```python
from build123d import *
from OCP.BRepFilletAPI import BRepFilletAPI_MakeChamfer

# Parameters (mm, degrees)
SKETCH1_W                = 70
SKETCH1_H                = 150
BOSS_EXTRUDE1_DEPTH      = 5
SKETCH2_W                = 4
SKETCH2_H                = 15
BOSS_EXTRUDE2_DEPTH      = 15
BOSS_EXTRUDE3_REACH      = 89.321
SKETCH3_R                = 3
CHAMFER1_SIZE            = 4
CHAMFER2_SIZE            = 4
CHAMFER3_SIZE            = 4
CHAMFER4_SIZE            = 10
CHAMFER5_SIZE            = 20
SKETCH4_W                = 3
SKETCH4_H                = 10
BOSS_EXTRUDE4_DEPTH      = 10
CHAMFER6_SIZE            = 2
SKETCH5_R                = 1.5
CUT_EXTRUDE1_DEPTH       = 100.969995499
CUT_EXTRUDE2_DEPTH       = 106
BOSS_EXTRUDE5_DEPTH      = 10
BOSS_EXTRUDE5_DEPTH_BACK = 3
SKETCH7_W                = 18
SKETCH7_H                = 2.192346064
CHAMFER7_SIZE            = 3
CHAMFER7_SIZE2           = 3.21710613
FILLET1_R                = 2
SKETCH8_R                = 1.5
CUT_EXTRUDE3_DEPTH       = 10
CHAMFER8_SIZE            = 1
CHAMFER8_SIZE2           = 0.487732589
FILLET2_R                = 1
SKETCH9_W                = 23.659390011
SKETCH9_H                = 22.018276252
CUT_EXTRUDE4_DEPTH       = 20


with BuildPart() as part:
    # Sketch1 → Boss-Extrude1 (new body)
    with BuildSketch(Plane(origin=(0, 0, 0), x_dir=(1, 0, 0), z_dir=(0, 1, 0))):
        Rectangle(SKETCH1_W, SKETCH1_H)
    extrude(amount=BOSS_EXTRUDE1_DEPTH)

    # Sketch2 → Boss-Extrude2 (add)
    with BuildSketch(Plane(origin=(0, 5, 0), x_dir=(1, 0, 0), z_dir=(0, 1, 0))):
        with Locations((-7, 62.5)):
            Rectangle(SKETCH2_W, SKETCH2_H)
        with Locations((7, 62.5)):
            Rectangle(SKETCH2_W, SKETCH2_H)
    extrude(amount=BOSS_EXTRUDE2_DEPTH)

    # Sketch3 → Boss-Extrude3 (add, up to next)
    with BuildSketch(Plane(origin=(-5, 0, 0), x_dir=(0, 0, -1), z_dir=(1, 0, 0)), mode=Mode.PRIVATE) as boss_extrude3_sk1:
        with Locations(Location((62.5, 12.5, 0), (0, 0, 180))):
            Circle(SKETCH3_R)
    boss_extrude3_tool1 = extrude(boss_extrude3_sk1.sketch, amount=BOSS_EXTRUDE3_REACH, mode=Mode.PRIVATE) - part.part
    add(boss_extrude3_tool1.solids().sort_by_distance((-5, 12.5, -62.5))[0])

    # Chamfer1
    chamfer1_edges = [part.edges().sort_by_distance(p)[0] for p in [
        (-7, 20, -70),
        (-7, 20, -55),
        (7, 20, -70),
        (7, 20, -55),
    ]]
    chamfer(chamfer1_edges, length=CHAMFER1_SIZE)

    # Chamfer2
    chamfer2_edges = [part.edges().sort_by_distance(p)[0] for p in [
        (-7, 5, -70),
        (-7, 5, -55),
        (7, 5, -70),
        (7, 5, -55),
    ]]
    chamfer(chamfer2_edges, length=CHAMFER2_SIZE)

    # Chamfer3
    chamfer3_edges = [part.edges().sort_by_distance(p)[0] for p in [
        (9, 5, -62.5),
        (-9, 5, -62.5),
    ]]
    chamfer(chamfer3_edges, length=CHAMFER3_SIZE)

    # Chamfer4
    chamfer4_edges = [part.edges().sort_by_distance(p)[0] for p in [
        (-35, 2.5, -75),
        (35, 2.5, -75),
    ]]
    chamfer(chamfer4_edges, length=CHAMFER4_SIZE)

    # Chamfer5
    chamfer5_edges = [part.edges().sort_by_distance(p)[0] for p in [
        (35, 2.5, 75),
        (-35, 2.5, 75),
    ]]
    chamfer(chamfer5_edges, length=CHAMFER5_SIZE)

    # Sketch4 → Boss-Extrude4 (add)
    with BuildSketch(Plane(origin=(0, 5, 0), x_dir=(1, 0, 0), z_dir=(0, 1, 0))):
        with Locations((26.5, -25)):
            Rectangle(SKETCH4_W, SKETCH4_H)
        with Locations((-26.5, -25)):
            Rectangle(SKETCH4_W, SKETCH4_H)
    extrude(amount=BOSS_EXTRUDE4_DEPTH)

    # Chamfer6
    chamfer6_edges = [part.edges().sort_by_distance(p)[0] for p in [
        (26.5, 15, 20),
        (26.5, 15, 30),
        (-26.5, 15, 20),
        (-26.5, 15, 30),
    ]]
    chamfer(chamfer6_edges, length=CHAMFER6_SIZE)

    # Sketch5 → Cut-Extrude1 (cut, through all)
    with BuildSketch(Plane(origin=(28, 0, 0), x_dir=(0, 0, -1), z_dir=(1, 0, 0))):
        with Locations((-25, 11)):
            Circle(SKETCH5_R)
    extrude(amount=-CUT_EXTRUDE1_DEPTH, mode=Mode.SUBTRACT)

    # Sketch6 → Cut-Extrude2 (cut)
    with BuildSketch(Plane(origin=(35, 0, 0), x_dir=(0, 0, -1), z_dir=(1, 0, 0))):
        Polygon((-75, 5), (44.602239444, 5), (44.602239444, 35.253881219), (84.386815395, 35.253881219), (84.386815395, 5), (84.386815395, -21.159404211), (-75, -21.159404211), align=None)
    extrude(amount=-CUT_EXTRUDE2_DEPTH, mode=Mode.SUBTRACT)


with BuildPart() as cut_extrude2_piece_1:
    # of the separate pieces the step leaves, piece 1, a body of its own (cut_extrude2_pieces)
    add(part.part.solids().sort_by_distance((-25, 13, 20))[0])

    # Sketch9 → Cut-Extrude4 (cut)
    with BuildSketch(Plane(origin=(0, 0, 16), x_dir=(-1, 0, 0), z_dir=(0, 0, -1))):
        with Locations((24.129769204, 9.145253251)):
            Rectangle(SKETCH9_W, SKETCH9_H)
    extrude(amount=-CUT_EXTRUDE4_DEPTH, mode=Mode.SUBTRACT)


with BuildPart() as cut_extrude2_piece_2:
    # of the separate pieces the step leaves, piece 2, a body of its own (cut_extrude2_pieces)
    add(part.part.solids().sort_by_distance((25, 13, 20))[0])

    # Sketch7 → Boss-Extrude5 (add, two sides: drawn at the far end of the back side and taken through both)
    with BuildSketch(Plane(origin=(28, 0, 0), x_dir=(0, 0, -1), z_dir=(1, 0, 0)).offset(-BOSS_EXTRUDE5_DEPTH_BACK)):
        with Locations((-25, 6.096173032)):
            Rectangle(SKETCH7_W, SKETCH7_H)
    extrude(amount=BOSS_EXTRUDE5_DEPTH + BOSS_EXTRUDE5_DEPTH_BACK)

    # Chamfer7: one chamfer whose edges measure the first distance from different faces: ONE call of the kernel's chamfer builder (chamfer() names one face for all edges)
    chamfer7_edges_1 = [cut_extrude2_piece_2.edges().sort_by_distance(p)[0] for p in [
        (25, 6.096173032, 34),
    ]]
    chamfer7_side_1 = [cut_extrude2_piece_2.faces().sort_by_distance(p)[0] for p in [
        (31.5, 6.096173032, 34),
    ]]
    chamfer7_edges_2 = [cut_extrude2_piece_2.edges().sort_by_distance(p)[0] for p in [
        (25, 6.096173032, 16),
    ]]
    chamfer7_side_2 = [cut_extrude2_piece_2.faces().sort_by_distance(p)[0] for p in [
        (25, 9.127734828, 25),
    ]]
    chamfer7 = BRepFilletAPI_MakeChamfer(cut_extrude2_piece_2.part.solid().wrapped)
    for e in chamfer7_edges_1:
        chamfer7.Add(CHAMFER7_SIZE, CHAMFER7_SIZE2, e.wrapped, chamfer7_side_1[0].wrapped)  # the first distance lies on this face
    for e in chamfer7_edges_2:
        chamfer7.Add(CHAMFER7_SIZE, CHAMFER7_SIZE2, e.wrapped, chamfer7_side_2[0].wrapped)  # the first distance lies on this face
    add(Compound.cast(chamfer7.Shape()), mode=Mode.REPLACE)

    # Fillet1
    fillet1_edges = [cut_extrude2_piece_2.edges().sort_by_distance(p)[0] for p in [
        (26.5, 7.192346064, 30),
        (26.5, 7.192346064, 20),
    ]]
    fillet(fillet1_edges, radius=FILLET1_R)

    # Sketch8 → Cut-Extrude3 (cut)
    with BuildSketch(Plane(origin=(0, 7.192346064, 0), x_dir=(1, 0, 0), z_dir=(0, 1, 0))):
        with Locations(Location((33.5, -20.5, 0), (0, 0, 270))):
            Circle(SKETCH8_R)
        with Locations(Location((33.5, -29.5, 0), (0, 0, 270))):
            Circle(SKETCH8_R)
    extrude(amount=-CUT_EXTRUDE3_DEPTH, mode=Mode.SUBTRACT)

    # Chamfer8
    chamfer8_edges = [cut_extrude2_piece_2.edges().sort_by_distance(p)[0] for p in [
        (33.5, 7.192346064, 19),
        (33.5, 7.192346064, 28),
    ]]
    chamfer8_side = [cut_extrude2_piece_2.faces().sort_by_distance(p)[0] for p in [
        (32.839348065, 7.192346064, 25.007845187),
    ]]
    chamfer(chamfer8_edges, length=CHAMFER8_SIZE, length2=CHAMFER8_SIZE2, reference=chamfer8_side[0])

    # Fillet2
    fillet2_edges = [cut_extrude2_piece_2.edges().sort_by_distance(p)[0] for p in [
        (38, 6.096173032, 34),
        (38, 6.096173032, 16),
    ]]
    fillet(fillet2_edges, radius=FILLET2_R)


solid = cut_extrude2_piece_2.part
```
Verification items for the finished model (mm, model axes). A direction names the side the tool comes from. Coordinates: 2 decimals unless noted, no trailing zeros. Write each loop counter-clockwise with the first axis right and the second up, starting at its lowest first coordinate (ties: lowest second). Pieces come first, ordered by that corner, then holes. Notation, with made-up numbers: M 75.5,47 L 91.5,47 A23 cw 91.5,61 Z; hole C 10.25,-2.5 d3. An arc over 180 degrees is marked long. Answer as a JSON object with one key per item and string values. Group by question number.
(1) Cross-section at D-D, the plane z = 25. Record the cut outline in (x, y).
(2) Cross-section at C-C, the plane y = 11. Record the cut outline in (x, z), and give its area (3 significant figures).
(3) Cross-section at B-B, the plane z = 29.5. Record the cut outline in (x, y), and give its area (3 significant figures).
(4) Material ranges on line 1 (X direction, y = 5.95, z = 29.5); line 2 (X direction, y = 10.75, z = 21.5); line 3 (Y direction, x = 31, z = 17.5), recorded low to high.
(5) Gauge pin test, flat ends, axial feed: pin 1 (2 mm diameter, centred on x = 28, z = 28.5, fed in from +Y); pin 2 (3.5 mm diameter, centred on x = 33.5, z = 24.5, fed in from +Y); pin 3 (6 mm diameter, centred on y = 12.5, z = 25.5, fed in from +X); pin 4 (0.9 mm diameter, centred on x = 26.5, y = 11.5, fed in from +Z). Record the tip position at first contact, or that the pin passes through.
(6) Cross-section at A-A, the plane x = 33.5. Record the cut outline in (y, z), and give its area (3 significant figures).
(7) Tool access check on faces 5 (the face through (32, 6, 34)), 6 (the face through (28, 9, 25)), 7 (the face through (26, 11, 30)). Record the directions out of +Z, -Z, +X, -X, +Y, -Y that give a thin tool (end or side, any length) a straight path to the whole face; none if there is none.
(8) Release check for a two-part mould opening along Z. For faces 1 (the face through (26, 11, 20)), 2 (the face through (25, 9, 25)), 3 (the face through (32.6, 5.9, 28.3)), 4 (the face through (26.52, 11.07, 26.5)) record: +Z half, -Z half, draft (parallel to the pull), parting line (faces both ways), or undercut.
Reply:
{
 "1": {"outline": "M 25,5 L 38,5 L 38,7.19 L 28,7.19 L 28,9.5 L 25,9.5 Z; M 25,12.5 L 28,12.5 L 28,15 L 25,15 Z"},
 "2": {"outline": "M 25,20 L 28,20 L 28,23.5 L 25,23.5 Z; M 25,26.5 L 28,26.5 L 28,30 L 25,30 Z", "area": "21.0 mm²"},
 "3": {"outline": "M 25,5 L 32,5 L 32,6.7 L 31,7.19 L 28,7.19 L 28,13.5 L 25,13.5 Z; M 35,5 L 38,5 L 38,7.19 L 36,7.19 L 35,6.7 Z", "area": "40.4 mm²"},
 "4": {"line 1": "25 to 32, 35 to 38", "line 2": "25 to 28", "line 3": "5 to 7.19"},
 "5": {"pin 1": "y = 15", "pin 2": "y = 7.19", "pin 3": "x = 28", "pin 4": "z = 30"},
 "6": {"outline": "M 5,16 L 7.19,16 L 7.19,18 L 6.7,19 L 5,19 Z; M 5,22 L 6.7,22 L 7.19,23 L 7.19,27 L 6.7,28 L 5,28 Z; M 5,31 L 6.7,31 L 7.19,32 L 7.19,34 L 5,34 Z", "area": "25.3 mm²"},
 "7": {"face 5": "+Z, +X, -X, +Y, -Y", "face 6": "+Z, -Z, +X, +Y", "face 7": "+Z, +X, -X, +Y"},
 "8": {"face 1": "-Z half", "face 2": "draft", "face 3": "undercut", "face 4": "undercut"}
}
